from build123d import *

# Parameters (mm, degrees)
F1_DEPTH = 18
F2_SIZE  = 5


with BuildPart() as f1:
    # F0 (on Front) → F1 (new body)
    with BuildSketch(Plane.XZ):
        Polygon((-9, 0), (-9, 20), (9, 20), (9, 0), (58, 0), (58, 40), (-58, 40), (-58, 0), align=None)
    extrude(amount=F1_DEPTH)

    # F2
    f2_edges = [f1.edges().sort_by_distance(p)[0] for p in [
        (-58, -9, 0),
        (58, -9, 0),
        (58, -9, 40),
        (-58, -9, 40),
    ]]
    chamfer(f2_edges, length=F2_SIZE)


solid = f1.part
For this review, take the finished solid that the model builds, in its own axes (mm). A direction names the side the tool comes from. Coordinates: 2 decimals unless noted, no trailing zeros. Loops run counter-clockwise (first coordinate to the right, second up) from the corner with the lowest first, then second, coordinate; pieces in that order, holes last. Notation, with made-up numbers: (-13, 56) - (21, 56) arc R19 cw to (21, 75) - close; hole circle Ø10 at (50, 85.5). An arc over 180 degrees is marked (long way). Use a Markdown table: item, result. Add a question column.
Item 1: We need section A-A (z = 13). Give the boundary of the cut face in (x, y).
Item 2: Mouldability with a two-part tool opening along X and no side actions: class faces 3 (the face through (58, -9, 20)), 4 (the face through (9, -9, 10)), 5 (the face through (-9, -9, 10)), 6 (the face through (-58, -9, 20)) as pulls with the +X half, pulls with the -X half, needs draft (parallel to the pull), parting line crosses it, or undercut.
Item 3: Tool access review of faces 1 (the face through (0, -9, 20)), 2 (the face through (55, -9, 38)): name each direction out of +Z, -Z, +X, -X, +Y, -Y from which nothing blocks a thin tool from reaching the whole face with its end or side.
Item 4: We need section B-B (y = -10.25). Give the boundary of the cut face in (x, z).
Item 5: Insertion check: pin 1 Ø8 at (x, z) = (32, 32.5) entering from +Y; pin 2 Ø5.5 at (x, y) = (-2, -6) entering from -Z. Each pin has a flat end and moves straight along its axis. Give the tip position at first contact, or say it passes through.
Item 6: For line 1 (X direction, y = -13.25, z = 17); line 2 (Z direction, x = -6.5, y = -10.25); line 3 (X direction, y = -2.75, z = 4), list the stretches that pass through material, from the lowest coordinate up.
Item 7: We need section C-C (x = -7.5). Give the boundary of the cut face in (y, z).
Results list:
| question | item | result |
|---|---|---|
| 1 | outline | (-58, -18) - (-9, -18) - (-9, 0) - (-58, 0) - close; (9, -18) - (58, -18) - (58, 0) - (9, 0) - close |
| 2 | face 3 | pulls with the +X half |
| 2 | face 4 | undercut |
| 2 | face 5 | undercut |
| 2 | face 6 | pulls with the -X half |
| 3 | face 1 | -Z, +Y, -Y |
| 3 | face 2 | +Z, +X, +Y, -Y |
| 4 | outline | (-58, 5) - (-53, 0) - (-9, 0) - (-9, 20) - (9, 20) - (9, 0) - (53, 0) - (58, 5) - (58, 35) - (53, 40) - (-53, 40) - (-58, 35) - close |
| 5 | pin 1 | stops at y = 0 |
| 5 | pin 2 | stops at z = 20 |
| 6 | line 1 | x = -58 to -9, 9 to 58 |
| 6 | line 2 | z = 20 to 40 |
| 6 | line 3 | x = -57 to -9, 9 to 57 |
| 7 | outline | (-18, 20) - (0, 20) - (0, 40) - (-18, 40) - close |
